Part model, mm, in its own coordinate system. A direction names the side the tool comes from. Coordinates: 2 decimals unless noted, no trailing zeros. Loops run counter-clockwise (first coordinate to the right, second up) from the corner with the lowest first, then second, coordinate; pieces in that order, holes last. Notation, with made-up numbers: (72, 75.25) - (111, 75.25) arc R31 cw to (111, 113.25) - close; hole circle Ø8 at (42.25, 15.5). An arc over 180 degrees is marked (long way). Answer as CSV lines item,"result".
from build123d import *

# Parameters (mm, degrees)
EXTRUDE_1_DEPTH = 4
SKETCH_2_R      = 3
EXTRUDE_2_DEPTH = 15
CHAMFER_1_SIZE  = 1


with BuildPart() as part:
    # Эскиз1 → Бобышка-Вытянуть1 (new body)
    with BuildSketch(Plane.XY):
        Polygon((5.773502692, 0), (2.886751346, 5), (-2.886751346, 5), (-5.773502692, 0), (-2.886751346, -5), (2.886751346, -5), align=None)
    extrude(amount=EXTRUDE_1_DEPTH)

    # Эскиз2 → Бобышка-Вытянуть2 (add)
    with BuildSketch(Plane(origin=(0, 0, 0), x_dir=(-1, 0, 0), z_dir=(0, 0, -1))):
        with Locations(Location((0, 0, 0), (0, 0, 180))):
            Circle(SKETCH_2_R)
    extrude(amount=EXTRUDE_2_DEPTH)

    # Фаска1
    chamfer_1_edges = [part.edges().sort_by_distance(p)[0] for p in [
        (-3, 0, -15),
    ]]
    chamfer(chamfer_1_edges, length=CHAMFER_1_SIZE)

    # Эскиз3 → Вырез-Повернуть1 (revolve, cut)
    with BuildSketch(Plane(origin=(0, 0, 0), x_dir=(1, 0, 0), z_dir=(0, 1, 0))):
        Polygon((-10.773502692, -0.651368439), (-4.973502692, -4), (-10.773502692, -4), align=None)
    revolve(axis=Axis((0, 0, 4), (0, 0, -1)), mode=Mode.SUBTRACT)


solid = part.part
Q1. Wall check: L1, parallel to Z at x = -2.5, y = 4; L2, parallel to Y at x = 0, z = -9.5; L3, parallel to Y at x = 0.75, z = -12. Give the ranges that are in metal, low to high.
Results:
L1,"z = 0 to 4"
L2,"y = -3 to 3"
L3,"y = -2.9 to 2.9"
Q2. Flat gauge pins, fed straight in: pin 1 (1 mm diameter, centred on x = 1, y = 2.5, fed in from -Z); pin 2 (2 mm diameter, centred on x = -3.5, y = -1, fed in from -Z). Where does each tip first touch, or does it go through?
Results:
pin 1,"stops at z = -14.81"
pin 2,"stops at z = -14.36"
Q3. Saw through at C-C (z = -1.5). Give the cut face in (x, y).
Results:
outline,"circle Ø6 at (0, 0)"
Q4. Saw through at B-B (z = 1.75). Give the cut face in (x, y).
Results:
outline,"(-5.77, 0) - (-2.89, -5) - (2.89, -5) - (5.77, 0) - (2.89, 5) - (-2.89, 5) - close"
Q5. Which spindle directions (+Z, -Z, +X, -X, +Y, -Y) get a long thin tool onto all of the face, cutting with end or side? Do faces 1 (the face through (0, 0, -15)), 2 (the face through (2.5, 2.3, 0)). Say none if no direction does.
Results:
face 1,"-Z, +X, -X, +Y, -Y"
face 2,"-Z"
